Work out the finished part from the listing and answer in its coordinate system (mm). Face numbers are marked on the shaded views. A direction names the side the tool comes from. Coordinates: 2 decimals unless noted, no trailing zeros. Order: outer loops, then holes, each group sorted by start corner. A loop starts at its lowest first (then second) coordinate and runs counter-clockwise, first axis right, second up. Notation, with made-up numbers: (63, -8) -> (115, -8) arc R27 ccw to (115, 31) -> close; hole circle Ø7 at (43.25, 32.5). An arc over 180 degrees is marked (long way). Write item = value, one per line. Start each with the question number.
Q1. Which of the six approach directions +Z, -Z, +X, -X, +Y, -Y give full straight-line access (tool end or side, diameter ignored) to the marked faces 1, 2, 3, 4 and 5?
Q2. The part is cut by section B-B, the plane y = 30. Determine the outline of the cut face in (x, z), plus the area to 3 significant figures.
Q3. For a pull along Y with two mould halves and no side action, classify the marked faces 6, 7, 8 and 9 as +Y half, -Y half, draft (parallel to the pull), parting line (faces both ways), or undercut.
Q4. The part is cut by section C-C, the plane z = -14.5. Determine the outline of the cut face in (x, y).
Q5. The part is cut by section D-D, the plane x = 2.5. Determine the outline of the cut face in (y, z).
Q6. Straight lines are drawn through the part: L1, parallel to X at y = 7.75, z = 0; L2, parallel to X at y = 12, z = 0; L3, parallel to X at y = 34.5, z = -12.5. For each, find the intervals that lie inside material, in ascending order. Write a range as from..to.
Q7. The part is cut by section A-A, the plane x = 17.5. Determine the outline of the cut face in (y, z), plus the area to 3 significant figures.
Q8. A flat-ended cylindrical pin translates along its axis: pin 1 (5 mm diameter, centred on y = 12, z = 12, fed in from -X). Find the tip coordinate at first contact, or state that the pin passes through.
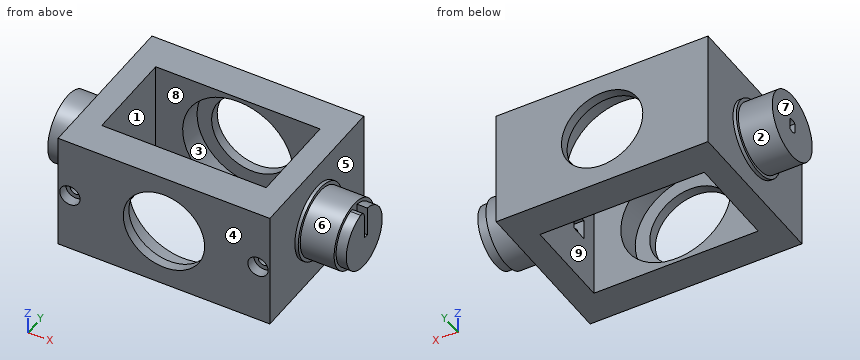
```python
from build123d import *

# Parameters (mm, degrees)
SKETCH_1_W          = 62.5
SKETCH_1_H          = 35
SKETCH_1_R          = 12
EXTRUDE_1_DEPTH     = 10
SKETCH_2_R          = 16.3
CUT_EXTRUDE_1_DEPTH = 7.2
SKETCH_4_W          = 7
SKETCH_4_H          = 35
EXTRUDE_3_DEPTH     = 37
SKETCH_5_R          = 3
CUT_EXTRUDE_3_DEPTH = 3
SKETCH_7_R          = 1.7
CUT_EXTRUDE_4_DEPTH = 20
SKETCH_9_W          = 6
SKETCH_9_H          = 5
CUT_EXTRUDE_5_DEPTH = 7
SKETCH_10_R         = 10
EXTRUDE_4_DEPTH     = 11
SKETCH_11_R         = 11
EXTRUDE_5_DEPTH     = 1
EXTRUDE_6_DEPTH     = 3
CUT_EXTRUDE_6_DEPTH = 5.5


with BuildPart() as part:
    # 草图1 → 凸台-拉伸1 (new body)
    with BuildSketch(Plane(origin=(0, 0, 0), x_dir=(1, 0, 0), z_dir=(0, 1, 0))):
        Rectangle(SKETCH_1_W, SKETCH_1_H)
        with Locations(Location((0, 0, 0), (0, 0, 270))):
            Circle(SKETCH_1_R, mode=Mode.SUBTRACT)
    extrude_1 = extrude(amount=EXTRUDE_1_DEPTH)

    # 草图2 → 切除-拉伸1 (cut)
    with BuildSketch(Plane(origin=(0, 10, 0), x_dir=(1, 0, 0), z_dir=(0, 1, 0))):
        with Locations(Location((0, 0, 0), (0, 0, 270))):
            Circle(SKETCH_2_R)
    cut_extrude_1 = extrude(amount=-CUT_EXTRUDE_1_DEPTH, mode=Mode.SUBTRACT)

    # 草图4 → 凸台-拉伸3 (add)
    with BuildSketch(Plane(origin=(0, 0, 0), x_dir=(1, 0, 0), z_dir=(0, 1, 0))):
        with Locations((27.75, 0)):
            Rectangle(SKETCH_4_W, SKETCH_4_H)
    extrude_3 = extrude(amount=EXTRUDE_3_DEPTH)

    # 草图5 → 切除-拉伸3 (cut)
    with BuildSketch(Plane(origin=(0, 0, 0), x_dir=(1, 0, 0), z_dir=(0, 1, 0))):
        with Locations(Location((27.75, 0, 0), (0, 0, 270))):
            Circle(SKETCH_5_R)
    cut_extrude_3 = extrude(amount=CUT_EXTRUDE_3_DEPTH, mode=Mode.SUBTRACT)

    # 草图7 → 切除-拉伸4 (cut)
    with BuildSketch(Plane(origin=(0, 0, 0), x_dir=(1, 0, 0), z_dir=(0, 1, 0))):
        with Locations(Location((27.75, 0, 0), (0, 0, 270))):
            Circle(SKETCH_7_R)
    cut_extrude_4 = extrude(amount=CUT_EXTRUDE_4_DEPTH, mode=Mode.SUBTRACT)

    # 草图9 → 切除-拉伸5 (cut)
    with BuildSketch(Plane(origin=(31.25, 0, 0), x_dir=(0, 0, -1), z_dir=(1, 0, 0))):
        with Locations((0, 17.5)):
            Rectangle(SKETCH_9_W, SKETCH_9_H)
    cut_extrude_5 = extrude(amount=-CUT_EXTRUDE_5_DEPTH, mode=Mode.SUBTRACT)

    # 镜向4: 凸台-拉伸3, 切除-拉伸3, 切除-拉伸4, 切除-拉伸5 across plane
    add(extrude_3.mirror(Plane.ZY))
    add(cut_extrude_3.mirror(Plane.ZY), mode=Mode.SUBTRACT)
    add(cut_extrude_4.mirror(Plane.ZY), mode=Mode.SUBTRACT)
    add(cut_extrude_5.mirror(Plane.ZY), mode=Mode.SUBTRACT)

    # 镜向5: 凸台-拉伸1, 切除-拉伸1 across plane
    add(extrude_1.mirror(Plane.ZX.offset(23.5)))
    add(cut_extrude_1.mirror(Plane.ZX.offset(23.5)), mode=Mode.SUBTRACT)

    # 草图10 → 凸台-拉伸4 (add)
    with BuildSketch(Plane(origin=(31.25, 0, 0), x_dir=(0, 0, -1), z_dir=(1, 0, 0))):
        with Locations(Location((0, 23.5, 0), (0, 0, 180))):
            Circle(SKETCH_10_R)
    extrude_4 = extrude(amount=EXTRUDE_4_DEPTH)

    # 草图11 → 凸台-拉伸5 (add)
    with BuildSketch(Plane(origin=(31.25, 0, 0), x_dir=(0, 0, -1), z_dir=(1, 0, 0))):
        with Locations(Location((0, 23.5, 0), (0, 0, 180))):
            Circle(SKETCH_11_R)
    extrude_5 = extrude(amount=EXTRUDE_5_DEPTH)

    # 镜向6: 凸台-拉伸4, 凸台-拉伸5 across plane
    add(extrude_4.mirror(Plane.ZY))
    add(extrude_5.mirror(Plane.ZY))

    # 草图12 → 凸台-拉伸6 (add)
    with BuildSketch(Plane(origin=(42.25, 0, 0), x_dir=(0, 0, -1), z_dir=(1, 0, 0))):
        with BuildLine():
            Line((0, 23.5), (-7.348469228, 23.5))
            ThreePointArc((-7.348469228, 23.5), (-8.510364232, 22.948683298), (-8.818163074, 21.7))
            ThreePointArc((-8.818163074, 21.7), (8.998706419, 23.652586976), (-8.874119675, 25))
            Line((-8.874119675, 25), (0, 25))
            Line((0, 25), (0, 23.5))
        make_face()
    extrude(amount=EXTRUDE_6_DEPTH)

    # 草图13 → 切除-拉伸6 (cut)
    with BuildSketch(Plane.ZY.offset(42.25)):
        with BuildLine():
            Line((-1.5612495, 24.75), (1.5612495, 24.75))
            ThreePointArc((1.5612495, 24.75), (2, 23.5), (1.5612495, 22.25))
            Line((1.5612495, 22.25), (-1.5612495, 22.25))
            ThreePointArc((-1.5612495, 22.25), (-2, 23.5), (-1.5612495, 24.75))
        make_face()
    extrude(amount=-CUT_EXTRUDE_6_DEPTH, mode=Mode.SUBTRACT)


solid = part.part
```
Model answer:
q1.face_1 = +Z, -Z
q1.face_2 = -X
q1.face_3 = none
q1.face_4 = +Z, -Z, +X, -X, -Y
q1.face_5 = +X
q2.outline = (-42.25, -7.6) -> (-32.25, -7.6) -> (-32.25, -8.87) -> (-31.25, -8.87) -> (-31.25, -17.5) -> (-24.25, -17.5) -> (-24.25, 17.5) -> (-31.25, 17.5) -> (-31.25, 8.87) -> (-32.25, 8.87) -> (-32.25, 7.6) -> (-42.25, 7.6) -> close; (24.25, -17.5) -> (31.25, -17.5) -> (31.25, -8.87) -> (32.25, -8.87) -> (32.25, -7.6) -> (42.25, -7.6) -> (42.25, -6.22) -> (45.25, -6.22) -> (45.25, 6.22) -> (42.25, 6.22) -> (42.25, 7.6) -> (32.25, 7.6) -> (32.25, 8.87) -> (31.25, 8.87) -> (31.25, 17.5) -> (24.25, 17.5) -> close
q2.area = 867 mm2
q3.face_6 = parting line
q3.face_7 = draft
q3.face_8 = undercut
q3.face_9 = undercut
q4.outline = (-31.25, 0) -> (31.25, 0) -> (31.25, 47) -> (-31.25, 47) -> close; hole (-24.25, 10) -> (-7.45, 10) -> (-7.45, 2.8) -> (7.45, 2.8) -> (7.45, 10) -> (24.25, 10) -> (24.25, 37) -> (7.45, 37) -> (7.45, 44.2) -> (-7.45, 44.2) -> (-7.45, 37) -> (-24.25, 37) -> close
q5.outline = (0, -17.5) -> (10, -17.5) -> (10, -16.11) -> (2.8, -16.11) -> (2.8, -11.74) -> (0, -11.74) -> close; (0, 11.74) -> (2.8, 11.74) -> (2.8, 16.11) -> (10, 16.11) -> (10, 17.5) -> (0, 17.5) -> close; (37, -17.5) -> (47, -17.5) -> (47, -11.74) -> (44.2, -11.74) -> (44.2, -16.11) -> (37, -16.11) -> close; (37, 16.11) -> (44.2, 16.11) -> (44.2, 11.74) -> (47, 11.74) -> (47, 17.5) -> (37, 17.5) -> close
q6.L1 = -31.25..-29.45, -26.05..-16.3, 16.3..26.05, 29.45..31.25
q6.L2 = -31.25..-29.45, -26.05..-24.25, 24.25..26.05, 29.45..31.25
q6.L3 = -31.25..-24.25, 24.25..31.25
q7.outline = (0, -17.5) -> (10, -17.5) -> (10, 17.5) -> (0, 17.5) -> close; (37, -17.5) -> (47, -17.5) -> (47, 17.5) -> (37, 17.5) -> close
q7.area = 700 mm2
q8.pin_1 = -31.25
